Model file for the job. Use its own axes, mm. Face numbers are marked on the shaded views. A direction names the side the tool comes from. Round coordinates to 2 decimals unless told otherwise and drop trailing zeros. Order: outer loops, then holes, each group sorted by start corner. A loop starts at its lowest first (then second) coordinate and runs counter-clockwise, first axis right, second up. Notation, with made-up numbers: (62.25, 28.25) - (71.25, 28.25) arc R16 ccw to (71.25, 52.25) - close; hole circle Ø3 at (84, 52). An arc over 180 degrees is marked (long way). Use one line per item in the form item = value.
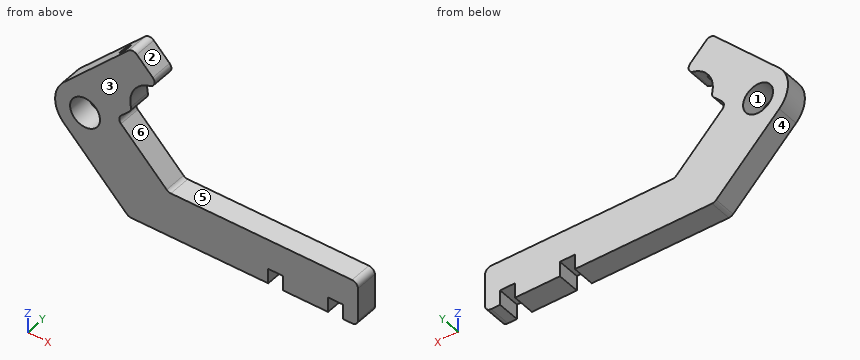
from build123d import *

# Parameters (mm, degrees)
F0_R     = 6.35
F1_DEPTH = 9.525
F2_R     = 2.38125
F3_DEPTH = 25.4
F4_R     = 2.54
F5_R     = 2.54


with BuildPart() as f1:
    # F0 (on Front) → F1 (new body)
    with BuildSketch(Plane.XZ):
        with BuildLine():
            ThreePointArc((20.258996, 9.87189), (22.492237, 21.066453), (33.413953, 24.386349))
            Line((33.413953, 24.386349), (20.62332, 37.176983))
            Line((20.62332, 37.176983), (-8.562513, 7.99115))
            ThreePointArc((-8.562513, 7.99115), (-12.282257, -0.989106), (-8.562513, -9.969362))
            Line((-8.562513, -9.969362), (18.922999, -37.454874))
            Line((18.922999, -37.454874), (78.158512, -37.454874))
            Line((78.158512, -37.454874), (78.158512, -31.104874))
            Line((78.158512, -31.104874), (84.508512, -31.104874))
            Line((84.508512, -31.104874), (84.508512, -37.454874))
            Line((84.508512, -37.454874), (103.558512, -37.454874))
            Line((103.558512, -37.454874), (103.558512, -31.104874))
            Line((103.558512, -31.104874), (109.908512, -31.104874))
            Line((109.908512, -31.104874), (109.908512, -37.454874))
            Line((109.908512, -37.454874), (116.258512, -37.454874))
            Line((116.258512, -37.454874), (116.258512, -18.404874))
            Line((116.258512, -18.404874), (35.794024, -18.404874))
            Line((35.794024, -18.404874), (13.888128, 3.501022))
            Line((13.888128, 3.501022), (20.258996, 9.87189))
        make_face()
        with Locations((0.417743, -0.989106)):
            Circle(F0_R, mode=Mode.SUBTRACT)
    extrude(amount=-F1_DEPTH)

    # F2 (on face) → F3 (cut)
    with BuildSketch(Plane(origin=(-8.276832, 0, 8.276832), x_dir=(0, -1, 0), z_dir=(-0.707107, 0, 0.707107))):
        with Locations((-4.7625, 31.345986)):
            Circle(F2_R)
    extrude(amount=-F3_DEPTH, mode=Mode.SUBTRACT)

    # F4
    f4_edges = [f1.edges().sort_by_distance(p)[0] for p in [
        (33.413953, 4.7625, 24.386349),
        (20.258996, 4.7625, 9.87189),
    ]]
    fillet(f4_edges, radius=F4_R)

    # F5
    f5_edges = [f1.edges().sort_by_distance(p)[0] for p in [
        (13.888128, 4.7625, 3.501022),
        (35.794024, 4.7625, -18.404874),
        (18.922999, 4.7625, -37.454874),
        (116.258512, 4.7625, -18.404874),
        (116.258512, 4.7625, -37.454874),
        (20.62332, 4.7625, 37.176983),
    ]]
    fillet(f5_edges, radius=F5_R)


solid = f1.part
(1) Slice it at D-D on z = -5. Give the cut face in (x, y) (3 decimals).
Report:
outline = (-11.632, 0) - (-4.505, 0) - (-4.505, 9.525) - (-11.632, 9.525) - close; (5.341, 0) - (22.389, 0) - (22.389, 9.525) - (5.341, 9.525) - close
(2) Slice it at C-C on x = 46. Give the cut face in (y, z) (3 decimals).
Report:
outline = (0, -37.455) - (9.525, -37.455) - (9.525, -18.405) - (0, -18.405) - close
(3) Tool access for the marked faces 4, 5 and 6: list every direction of +Z, -Z, +X, -X, +Y, -Y with a clear straight run to the whole face (end or side of a thin tool).
Report:
face_4 = -Z, -X, +Y, -Y
face_5 = +Z, +X, +Y, -Y
face_6 = +X, +Y, -Y
(4) Slice it at A-A on y = 3.75. Count the separate pieces of the cut face and the enclosed holes in it, then the cut area to 3 significant figures.
Report:
separate_pieces = 2
enclosed_holes = 1
area = 3,130 mm2
(5) Pull direction X, two halves, no side cores. Call the marked faces 1, 2 and 3: released by +X, released by -X, zero draft, split by the parting line, or undercut.
Report:
face_1 = undercut
face_2 = released by +X
face_3 = zero draft
(6) Pin check, flat tips, straight feed: pin 1 (8 mm diameter, centred on x = 17.5, z = 15, fed in from -Y); pin 2 (1.9 mm diameter, centred on y = 4.5, z = -36, fed in from -X); pin 3 (5 mm diameter, centred on x = 29.5, y = 5.5, fed in from +Z); pin 4 (1.9 mm diameter, centred on y = 5.5, z = -34.5, fed in from -X). Stop position of each tip, or through.
Report:
pin_1 = 0
pin_2 = 16.52
pin_3 = 30.8
pin_4 = 15.02
(7) Probe probe 1 along Z at (x, y) = (83, 8.5); probe 2 along Z at (x, y) = (61.5, 6.5); probe 3 along Z at (x, y) = (0, 8.25). List the from-to ranges inside material, lowest first. Write a range as [from, to].
Report:
probe_1 = [-31.1, -18.4]
probe_2 = [-37.45, -18.4]
probe_3 = [-18.53, -7.33], [5.35, 16.55]
(8) Slice it at B-B on z = 3. Give the cut face in (x, y) (1 decimal).
Report:
outline = (-11.6, 0) - (-4.5, 0) - (-4.5, 9.5) - (-11.6, 9.5) - close; (5.4, 0) - (15, 0) - (15, 9.5) - (5.4, 9.5) - close
